Could you check a few things on this drawing? It's one solid part, dimensions in mm from its lowest x, y, z. A direction names the side the tool comes from. Round coordinates to 2 decimals unless told otherwise and drop trailing zeros. Loops run counter-clockwise (first coordinate to the right, second up) from the corner with the lowest first, then second, coordinate; pieces in that order, holes last. Notation, with made-up numbers: M -32,81.5 L 7,81.5 A31 cw 7,105.5 Z; hole C -31.5,68.5 d10. An arc over 180 degrees is marked long. Return JSON: item names as keys, results as strings.
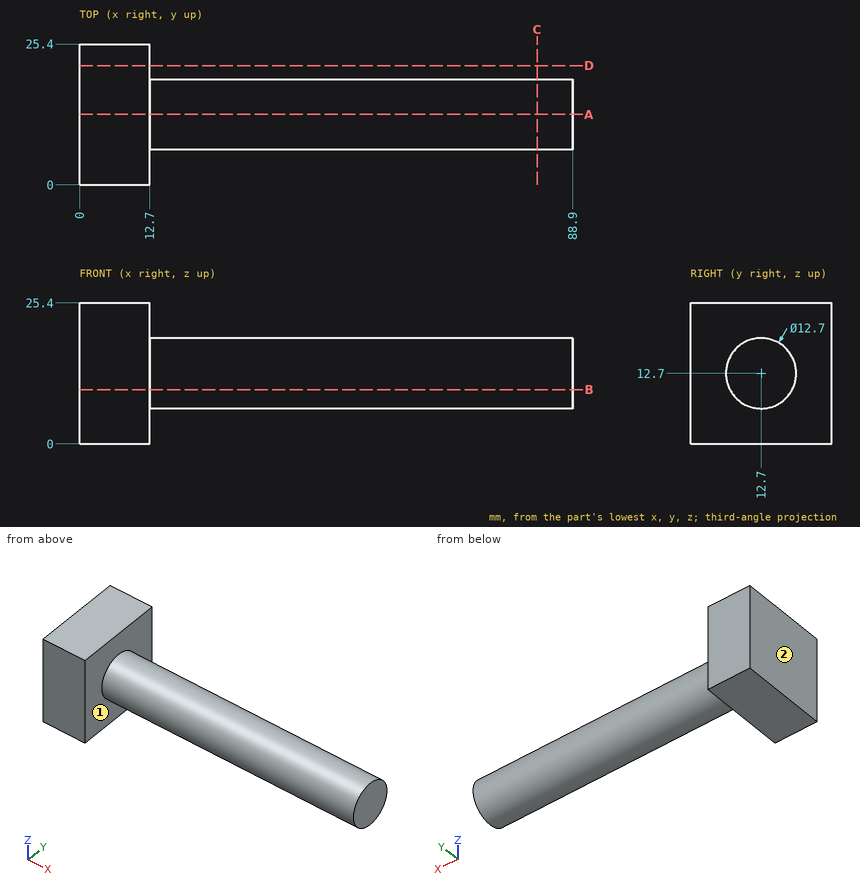
Q1. Suppose I cut it at D-D, the plane y = 21.5. Please give me the cut outline in (x, z), plus the area to 3 significant figures.
Results:
{"outline": "M 0,0 L 12.7,0 L 12.7,25.4 L 0,25.4 Z", "area": "323 mm2"}
Q2. Suppose I cut it at A-A, the plane y = 12.7. Please give me the cut outline in (x, z), plus the area to 3 significant figures.
Results:
{"outline": "M 0,0 L 12.7,0 L 12.7,6.35 L 88.9,6.35 L 88.9,19.05 L 12.7,19.05 L 12.7,25.4 L 0,25.4 Z", "area": "1,290 mm2"}
Q3. On a 3-axis mill with a long thin cutter (end or side, diameter ignored), from which of +Z, -Z, +X, -X, +Y, -Y can I reach the whole of each face in a straight line? I mean the marked faces 1 and 2. Say none if no direction works.
Results:
{"face 1": "+X", "face 2": "+Z, -Z, -X, +Y, -Y"}
Q4. Suppose I cut it at B-B, the plane z = 9.75. Please give me the cut outline in (x, y), plus the area to 3 significant figures.
Results:
{"outline": "M 0,0 L 12.7,0 L 12.7,7.08 L 88.9,7.08 L 88.9,18.32 L 12.7,18.32 L 12.7,25.4 L 0,25.4 Z", "area": "1,180 mm2"}
Q5. If I drill on line 1 along X through (y, z) = (5.5, 21.25); line 2 along Z through (x, y) = (60, 12.75); line 3 along Y through (x, z) = (82, 10.5), over which ranges is the centre line in solid material (lowest first)?
Results:
{"line 1": "x = 0 to 12.7", "line 2": "z = 6.35 to 19.05", "line 3": "y = 6.74 to 18.66"}
Q6. Suppose I cut it at C-C, the plane x = 82.5. Please give me the cut outline in (y, z).
Results:
{"outline": "C 12.7,12.7 d12.7"}
Q7. I'm going to push flat-ended pins straight in: pin 1 Ø12 at (x, y) = (38.5, 19) entering from +Z; pin 2 Ø5 at (x, z) = (68.5, 16) entering from -Y; pin 3 Ø1 at (x, y) = (62, 5) entering from +Z; pin 4 Ø2 at (x, z) = (67.5, 12.5) entering from +Y. Where does each tip first touch, or does it pass through?
Results:
{"pin 1": "stops at z = 19.04", "pin 2": "stops at y = 6.4", "pin 3": "passes through", "pin 4": "stops at y = 19.05"}
